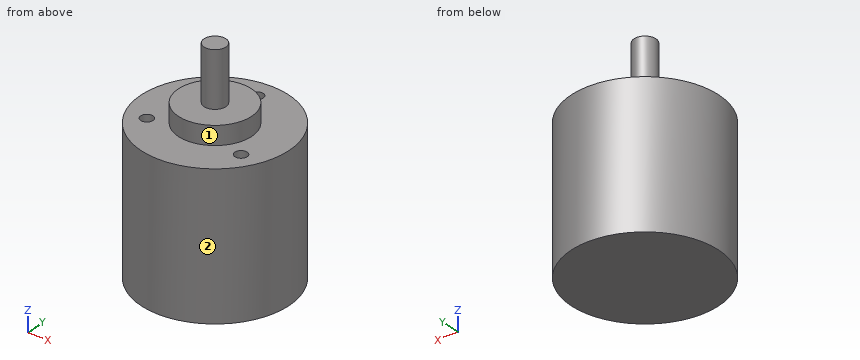
from build123d import *

# Parameters (mm, degrees)
SKETCH1_R                = 20.2311
BOSS_EXTRUDE1_DEPTH      = 19.5199
SKETCH2_R                = 10.0203
BOSS_EXTRUDE2_DEPTH      = 5.08
SKETCH3_R                = 3.00355
BOSS_EXTRUDE3_DEPTH      = 15.0241
M3_CLEARANCE_HOLE1_D     = 3.4
M3_CLEARANCE_HOLE1_DEPTH = 7.0000114
M3_CLEARANCE_HOLE1_TIP   = 1.021463052


with BuildPart() as part:
    # Sketch1 → Boss-Extrude1 (new, symmetric)
    with BuildSketch(Plane.XY):
        Circle(SKETCH1_R)
    extrude(amount=BOSS_EXTRUDE1_DEPTH, both=True)

    # Sketch2 → Boss-Extrude2 (add)
    with BuildSketch(Plane.XY.offset(19.5199)):
        Circle(SKETCH2_R)
    extrude(amount=BOSS_EXTRUDE2_DEPTH)

    # Sketch3 → Boss-Extrude3 (add)
    with BuildSketch(Plane.XY.offset(24.5999)):
        Circle(SKETCH3_R)
    extrude(amount=BOSS_EXTRUDE3_DEPTH)

    # M3 Clearance Hole1
    with Locations(Plane.XY.offset(19.5199)):
        with Locations((0, 15), (12.990381057, -7.5), (-12.990381057, -7.5)):
            Hole(M3_CLEARANCE_HOLE1_D / 2, depth=M3_CLEARANCE_HOLE1_DEPTH)
            with Locations((0, 0, -(M3_CLEARANCE_HOLE1_DEPTH + M3_CLEARANCE_HOLE1_TIP / 2))):  # 118° drill point
                Cone(0, M3_CLEARANCE_HOLE1_D / 2, M3_CLEARANCE_HOLE1_TIP, mode=Mode.SUBTRACT)


solid = part.part
Build history of the part. All positions in model axes, mm. Face numbers are marked on the shaded views. A direction names the side the tool comes from. Coordinates: 2 decimals unless noted, no trailing zeros. Write each loop counter-clockwise with the first axis right and the second up, starting at its lowest first coordinate (ties: lowest second). Pieces come first, ordered by that corner, then holes. Notation, with made-up numbers: (-0.75, -2) -> (23.25, -2) arc R23 cw to (23.25, 29) -> close; hole circle Ø5 at (-22, -4.5). An arc over 180 degrees is marked (long way). Use CSV: the item, a comma, the result in double quotes. Start each with the question number.
Q1. Drill centre lines: probe 1 along Y at (x, z) = (0, 17.75); probe 2 along Z at (x, y) = (-10.5, -1.5); probe 3 along Z at (x, y) = (-7, -4.5). Where is each one in solid material? Low to high.
Q2. Cut at C-C, the plane y = 6.5. List the corners of the cut face in (x, z).
Q3. Flat gauge pins, fed straight in: pin 1 Ø4 at (x, y) = (12.99, -7.5) entering from +Z; pin 2 Ø4 at (x, z) = (3, 33) entering from -Y; pin 3 Ø2 at (x, z) = (-1.5, 18) entering from +Y. Where does each tip first touch, or does it go through?
Q4. Cut at A-A, the plane y = 0. List the corners of the cut face in (x, z), then the cut area to 3 significant figures.
Q5. Cut at B-B, the plane z = 34.5. List the corners of the cut face in (x, y), then the cut area to 3 significant figures.
Q6. Cut at D-D, the plane z = -13.5. List the corners of the cut face in (x, y), then the cut area to 3 significant figures.
Q7. 3-axis set-ups, long thin cutter, end or side, ignore diameter. For the marked faces 1 and 2: which of +Z, -Z, +X, -X, +Y, -Y reach the whole face in a straight line?
Checked values:
1,probe 1,"y = -20.23 to 13.3, 16.7 to 20.23"
1,probe 2,"z = -19.52 to 19.52"
1,probe 3,"z = -19.52 to 24.6"
2,outline,"(-19.16, -19.52) -> (19.16, -19.52) -> (19.16, 19.52) -> (7.63, 19.52) -> (7.63, 24.6) -> (-7.63, 24.6) -> (-7.63, 19.52) -> (-19.16, 19.52) -> close"
3,pin 1,"stops at z = 19.52"
3,pin 2,"stops at y = -2.83"
3,pin 3,"stops at y = 20.22"
4,outline,"(-20.23, -19.52) -> (20.23, -19.52) -> (20.23, 19.52) -> (10.02, 19.52) -> (10.02, 24.6) -> (3, 24.6) -> (3, 39.62) -> (-3, 39.62) -> (-3, 24.6) -> (-10.02, 24.6) -> (-10.02, 19.52) -> (-20.23, 19.52) -> close"
4,area,"1,770 mm²"
5,outline,"circle Ø6.01 at (0, 0)"
5,area,"28.3 mm²"
6,outline,"circle Ø40.46 at (0, 0)"
6,area,"1,290 mm²"
7,face 1,"+Z"
7,face 2,"+Z, -Z"
